```python
from build123d import *

# Parameters (mm, degrees)
SKETCH1_R                    = 9.525
EXTRUDE1_DEPTH               = 304.8
CHAMFER1_SIZE                = 0.79375
F_5_16_18_TAPPED_HOLE1_D     = 6.5278
F_5_16_18_TAPPED_HOLE1_DEPTH = 24.6063008
F_5_16_18_TAPPED_HOLE1_TIP   = 1.961148974
CUT_EXTRUDE1_DEPTH           = 12.7


with BuildPart() as part:
    # Sketch1 → Extrude1 (new body)
    with BuildSketch(Plane.XY):
        with Locations(Location((0, 0, 0), (0, 0, 180))):
            Circle(SKETCH1_R)
    extrude(amount=EXTRUDE1_DEPTH)

    # Chamfer1
    chamfer1_edges = [part.edges().sort_by_distance(p)[0] for p in [
        (9.525, 0, 0),
        (9.525, 0, 304.8),
    ]]
    chamfer(chamfer1_edges, length=CHAMFER1_SIZE)

    # 5/16-18 Tapped Hole1
    with Locations(Plane.XY.offset(304.8)):
        with Locations((0, 0)):
            Hole(F_5_16_18_TAPPED_HOLE1_D / 2, depth=F_5_16_18_TAPPED_HOLE1_DEPTH)
            with Locations((0, 0, -(F_5_16_18_TAPPED_HOLE1_DEPTH + F_5_16_18_TAPPED_HOLE1_TIP / 2))):  # 118° drill point
                Cone(0, F_5_16_18_TAPPED_HOLE1_D / 2, F_5_16_18_TAPPED_HOLE1_TIP, mode=Mode.SUBTRACT)

    # Sketch4 → Cut-Extrude1 (cut)
    with BuildSketch(Plane(origin=(0, 0, 0), x_dir=(-1, 0, 0), z_dir=(0, 0, -1))):
        with BuildLine():
            Line((-7.9375, 5.265141855), (-7.9375, -5.265141855))
            ThreePointArc((-7.9375, -5.265141855), (-9.525, 0), (-7.9375, 5.265141855))
        make_face()
        with BuildLine():
            Line((7.9375, 5.265141855), (7.9375, -5.265141855))
            ThreePointArc((7.9375, -5.265141855), (9.525, 0), (7.9375, 5.265141855))
        make_face()
    extrude(amount=-CUT_EXTRUDE1_DEPTH, mode=Mode.SUBTRACT)


solid = part.part
```
Build history of the part. All positions in model axes, mm. A direction names the side the tool comes from. Round coordinates to 2 decimals unless told otherwise and drop trailing zeros. Write each loop counter-clockwise with the first axis right and the second up, starting at its lowest first coordinate (ties: lowest second). Pieces come first, ordered by that corner, then holes. Notation, with made-up numbers: (12.5, -33.5) - (17.5, -33.5) arc R27 ccw to (17.5, -16.5) - close; hole circle Ø5 at (-22, 75.5). An arc over 180 degrees is marked (long way). Write each question's results on one line, items separated by ' | '. Start each with the question number.
Item 1: Saw through at A-A (z = 19). Write the cut outline in (x, y) (3 decimals).
Item 2: Mould opens along X. For faces 1 (the face through (0, 0, 0)), 2 (the face through (-8.8, 3.65, 150.28)), 3 (the face through (0.708, -3.186, 292.325)) say: pulls with the +X half, pulls with the -X half, needs draft (parallel to the pull), parting line crosses it, or undercut.
Item 3: Wall check: L1, parallel to Y at x = 0, z = 287.75 (3 decimals); L2, parallel to Y at x = 0.25, z = 157.5; L3, parallel to X at y = -5.25, z = 117.5. Give the ranges that are in metal, low to high. Write a range as [from, to].
Item 4: Which spindle directions (+Z, -Z, +X, -X, +Y, -Y) get a long thin tool onto all of the face, cutting with end or side? Do faces 4 (the face through (-7.938, 0, 6)), 5 (the face through (7.938, 0, 6)), 6 (the face through (0.14, 8.86, 0.13)). Say none if no direction does.
Item 5: Drop flat-ended pins along their axis: P1, Ø0.8, axis at x = 8.5, y = -0.5, coming from the -Z side; P2, Ø8, axis at y = -6, z = 266.5, coming from the -X side; P3, Ø2, axis at y = -3, z = 69, coming from the +X side. Give the stop position or say it passes through.
Results are:
1) outline: circle Ø19.05 at (0, 0)
2) face 1: needs draft | face 2: parting line crosses it | face 3: undercut
3) L1: y = [-9.525, -3.264], [3.264, 9.525] | L2: y = [-9.52, 9.52] | L3: x = [-7.95, 7.95]
4) face 4: -Z, -X, +Y, -Y | face 5: -Z, +X, +Y, -Y | face 6: -Z, +Y
5) P1: stops at z = 12.7 | P2: stops at x = -9.31 | P3: stops at x = 9.31
